Input: part model. Units: mm. Frame: model coordinates. A direction names the side the tool comes from. Coordinates: 2 decimals unless noted, no trailing zeros. Order: outer loops, then holes, each group sorted by start corner. A loop starts at its lowest first (then second) coordinate and runs counter-clockwise, first axis right, second up. Notation, with made-up numbers: M 35.25,-6.5 L 66.25,-6.5 A25 ccw 66.25,31.5 Z; hole C -0.5,50.25 d3. An arc over 180 degrees is marked long. Answer in a Markdown table with one row per item.
Autodesk Inventor part; units mm, degrees
ref_plane "YZ Plane" through (0, 0, 0) normal (1, 0, 0) x (0, 1, 0)
ref_plane "XZ Plane" through (0, 0, 0) normal (0, 1, 0) x (-1, 0, 0)
ref_plane "XY Plane" through (0, 0, 0) normal (0, 0, 1) x (1, 0, 0)
sketch "Sketch1" plane through (0, 0, 0) normal (0, 0, 1) x (1, 0, 0)
  circle A0 centre (0, 0) radius 6
  dimension "d0" = 12
extrude "Extrusion1" add sketch "Sketch1" along normal mid plane 43.3
thread "Thread1"
sketch "Sketch2" plane through (0, 0, 21.65) normal (0, 0, 1) x (1, 0, 0)
  circle A0 centre (0, 0) radius 5.22
  dimension "d5" = 10.44
extrude "Extrusion2" add sketch "Sketch2" along normal blind 5
fillet "Fillet1" radius 0.2 1 edges at (-5.22, 0, 26.65)
fillet "Fillet2" radius 0.2 1 edges at (-5.22, 0, 21.65)
sketch "Sketch3" plane through (0, 0, -21.65) normal (0, 0, -1) x (-1, 0, 0)
  circle A0 centre (0, 0) radius 5.58
  dimension "d10" = 11.16
extrude "Extrusion3" add sketch "Sketch3" along normal blind 12.65
sketch "Sketch4" plane through (0, 0, -34.3) normal (0, 0, -1) x (-1, 0, 0)
  circle A0 centre (0, 2.2194) radius 2.7
  point P0 (0, 0)
  dimension "d13" = 5.4
extrude "Extrusion4" add sketch "Sketch4" along normal blind 4.5
draft "FaceDraft1" angle 5 pull direction (0, 0, -1) faces at (-2.6912, 2.0021, -37.3) fixed edges at (2.7, 2.2194, -34.3)
sketch "Sketch5" plane through (0, 0, -34.3) normal (0, 0, -1) x (-1, 0, 0)
  circle A0 centre (0, -3.4527) radius 1.2802
  point P0 (0, 0)
extrude "Extrusion5" add sketch "Sketch5" along normal blind 1.56
fillet "Fillet3" radius 1.2 1 edges at (1.2802, -3.4527, -35.86)
properties part number "LJ12A3-4-z-BY inductive switch"
1) Contact query for flat-ended pins moving along their axis: pin 1 (3.5 mm diameter, centred on x = 2.5, y = -1.5, fed in from -Z); pin 2 (2 mm diameter, centred on y = 2, z = -22.5, fed in from +X); pin 3 (1 mm diameter, centred on y = -3.5, z = 14, fed in from +X). Output: stop coordinate, or through.
Resolved:
| item | result |
|---|---|
| pin 1 | stops at z = -34.3 |
| pin 2 | stops at x = 5.82 |
| pin 3 | stops at x = 5.2 |
2) Mould query, pull axis Y, two halves, no side actions, for faces 1 (the face through (0.17, -4.72, -34.48)), 2 (the face through (-6, 0, 0)), 3 (the face through (0, 2, -38.8)). Classes: +Y half, -Y half, draft (parallel to the pull), parting line (faces both ways), or undercut.
Resolved:
| item | result |
|---|---|
| face 1 | undercut |
| face 2 | parting line |
| face 3 | draft |
3) Reachability of faces 4 (the face through (-3, -5, 21.65)), 5 (the face through (0, 0, 26.65)), 6 (the face through (0, -1, -34.3)) from +Z, -Z, +X, -X, +Y, -Y: full face, straight path, thin tool, end or side. Return the list, or none.
Resolved:
| item | result |
|---|---|
| face 4 | +Z |
| face 5 | +Z, +X, -X, +Y, -Y |
| face 6 | -Z |
4) Material intervals for probe 1 along Z at (x, y) = (3.75, 2); probe 2 along Y at (x, z) = (-2, -25); probe 3 along Z at (x, y) = (4, -4), sorted ascending.
Resolved:
| item | result |
|---|---|
| probe 1 | z = -34.3 to 26.65 |
| probe 2 | y = -5.21 to 5.21 |
| probe 3 | z = -21.65 to 21.65 |
5) Cut plane A-A, the plane z = -9.5. Output: boundary loops of the cut face in (x, y), and give its area (3 significant figures).
Resolved:
| item | result |
|---|---|
| outline | C 0,0 d12 |
| area | 113 mm2 |
